from build123d import *

# Parameters (mm, degrees)
FILLET1_R   = 1.27
HEX_2_DEPTH = 12


with BuildPart() as part:
    # BodySke → Base-Revolve (revolve)
    with BuildSketch(Plane.XY, mode=Mode.PRIVATE) as base_revolve_sk:
        Polygon((0, 0), (0, 15.6), (2.4, 18), (24, 18), (24, 12), (92.352, 12), (94, 10.352), (94, 0), align=None)
    revolve(base_revolve_sk.sketch.rotate(Axis((-31.75, 0, 0), (1, 0, 0)), 90), axis=Axis((-31.75, 0, 0), (1, 0, 0)))  # turned: the seam where the file's is

    # Fillet1
    fillet1_edges = [part.edges().sort_by_distance(p)[0] for p in [
        (24, 0, -12),
    ]]
    fillet(fillet1_edges, radius=FILLET1_R)

    # Sketch2 → Hex-PreBroach (revolve, cut)
    with BuildSketch(Plane.XY, mode=Mode.PRIVATE) as hex_prebroach_sk:
        Polygon((0, 9.5), (12, 9.5), (17.484827557, 0), (0, 0), align=None)
    revolve(hex_prebroach_sk.sketch.rotate(Axis((0, 0, 0), (1, 0, 0)), 90), axis=Axis((0, 0, 0), (1, 0, 0)), mode=Mode.SUBTRACT)  # turned: the seam where the file's is

    # Sketch3 → Hex 2 (cut)
    with BuildSketch(Plane(origin=(0, 0, 0), x_dir=(0, 0.5, 0.866025404), z_dir=(-1, 0, 0))):
        Polygon((5.484827557, 9.5), (-5.484827557, 9.5), (-10.969655115, 0), (-5.484827557, -9.5), (5.484827557, -9.5), (10.969655115, 0), align=None)
    extrude(amount=-HEX_2_DEPTH, mode=Mode.SUBTRACT)


solid = part.part
Here's how the part is built. I have some questions about the finished solid (model axes, mm). A direction names the side the tool comes from. Coordinates: 2 decimals unless noted, no trailing zeros. Write each loop counter-clockwise with the first axis right and the second up, starting at its lowest first coordinate (ties: lowest second). Pieces come first, ordered by that corner, then holes.
Item 1: If I drill on line 1 (X direction, y = 2.5, z = 13); line 2 (X direction, y = -7, z = -2); line 3 (Y direction, x = 5, z = -1), over which ranges is the centre line in solid material (lowest first)?
Item 2: If we mould it in two halves opening along Y, with no side actions, what happens to faces 4 (the flat face through (5.916, -8.266, 4.683)), 5 (the flat face through (94, 0, 0)), 6 (the cylindrical face through (13.351, -12.165, -13.267))? For each: +Y half, -Y half, draft (parallel to the pull), parting line (faces both ways), or undercut.
Item 3: On a 3-axis mill with a long thin cutter (end or side, diameter ignored), from which of +Z, -Z, +X, -X, +Y, -Y can I reach the whole of each face in a straight line? I mean faces 1 (the flat face through (5.9, 8.2, 4.8)), 2 (the flat face through (24, 11, -8)), 3 (the flat face through (0, 0, -10)). Say none if no direction works.
Item 4: I want a section at A-A on x = 26.5. Write out the boundary of the cut face in (y, z), and give its area (3 significant figures).
Item 5: Will these pins go through, and if not, where does the flat tip stop? pin 1 (10 mm diameter, centred on x = 43, z = 8, fed in from +Y); pin 2 (10 mm diameter, centred on x = 66, z = 0, fed in from +Y); pin 3 (5 mm diameter, centred on y = -4.5, z = 6, fed in from -X).
Findings below:
1. line 1: x = 0 to 24
1. line 2: x = 13.28 to 94
1. line 3: y = -17.97 to -10.39, 10.39 to 17.97
2. face 4: undercut
2. face 5: draft
2. face 6: parting line
3. face 1: -X
3. face 2: +X
3. face 3: +Z, -Z, -X, +Y, -Y
4. outline: circle Ø24 at (0, 0)
4. area: 452 mm2
5. pin 1: stops at y = 11.62
5. pin 2: stops at y = 12
5. pin 3: stops at x = 12
